```python
from build123d import *

# Parameters (mm, degrees)
F0_W     = 38.1
F0_H     = 19.05
F1_DEPTH = 19.05
F2_W     = 19.05
F2_H     = 19.05
F3_DEPTH = 38.1
F4_W     = 19.05
F4_H     = 19.05
F5_DEPTH = 19.05


with BuildPart() as f1:
    # F0 (on Top) → F1 (new body)
    with BuildSketch(Plane.XY):
        with Locations((19.05, 9.525)):
            Rectangle(F0_W, F0_H)
    extrude(amount=F1_DEPTH)

    # F2 (on face) → F3 (join)
    with BuildSketch(Plane.XY.offset(19.05)):
        with Locations((28.575, 9.525)):
            Rectangle(F2_W, F2_H)
    extrude(amount=F3_DEPTH)

    # F4 (on face) → F5 (join)
    with BuildSketch(Plane(origin=(0, 19.05, 0), x_dir=(-1, 0, 0), z_dir=(0, 1, 0))):
        with Locations((-28.575, 47.625)):
            Rectangle(F4_W, F4_H)
    extrude(amount=F5_DEPTH)


solid = f1.part
```
Check sheet for the modelled part. Datum: model origin and axes. Units: mm. A direction names the side the tool comes from. Round coordinates to 2 decimals unless told otherwise and drop trailing zeros. Order: outer loops, then holes, each group sorted by start corner. A loop starts at its lowest first (then second) coordinate and runs counter-clockwise, first axis right, second up. Notation, with made-up numbers: (26, 63) -> (75, 63) arc R24 ccw to (75, 79) -> close; hole circle Ø9 at (-39.75, -10.5). An arc over 180 degrees is marked (long way). Use CSV: the item, a comma, the result in double quotes.
(1) Depth check by flat-ended pin: pin 1 (1 mm diameter, centred on y = 6.5, z = 32, fed in from -X); pin 2 (10 mm diameter, centred on x = 16, y = 32.5, fed in from -Z); pin 3 (12 mm diameter, centred on x = 10.5, y = 14.5, fed in from -Z); pin 4 (9.5 mm diameter, centred on x = 12, y = 13, fed in from +Z). Enter the tip coordinate at first touch or a pass-through.
Worked out:
pin 1,"x = 19.05"
pin 2,"z = 38.1"
pin 3,"z = 0"
pin 4,"z = 19.05"
(2) Cross-section at B-B (y = 13). Record the boundary of the cut face in (x, z).
Worked out:
outline,"(0, 0) -> (38.1, 0) -> (38.1, 57.15) -> (19.05, 57.15) -> (19.05, 19.05) -> (0, 19.05) -> close"
(3) Cross-section at C-C (z = 28). Record the boundary of the cut face in (x, y).
Worked out:
outline,"(19.05, 0) -> (38.1, 0) -> (38.1, 19.05) -> (19.05, 19.05) -> close"
(4) Material ranges on line 1 along Z through (x, y) = (25, 24); line 2 along Z through (x, y) = (3, 18), recorded low to high. Write a range as from..to.
Worked out:
line 1,"38.1..57.15"
line 2,"0..19.05"
(5) Tool access check on faces 1 (the face through (19.05, 15, 42)), 2 (the face through (29, 38.1, 48)), 3 (the face through (29, 28, 38.1)). Record the directions out of +Z, -Z, +X, -X, +Y, -Y that give a thin tool (end or side, any length) a straight path to the whole face; none if there is none.
Worked out:
face 1,"+Z, -X, +Y, -Y"
face 2,"+Z, -Z, +X, -X, +Y"
face 3,"-Z, +X, -X, +Y"
(6) Cross-section at A-A (x = 30.5). Record the boundary of the cut face in (y, z).
Worked out:
outline,"(0, 0) -> (19.05, 0) -> (19.05, 38.1) -> (38.1, 38.1) -> (38.1, 57.15) -> (0, 57.15) -> close"
(7) Cross-section at D-D (x = 6). Record the boundary of the cut face in (y, z).
Worked out:
outline,"(0, 0) -> (19.05, 0) -> (19.05, 19.05) -> (0, 19.05) -> close"
